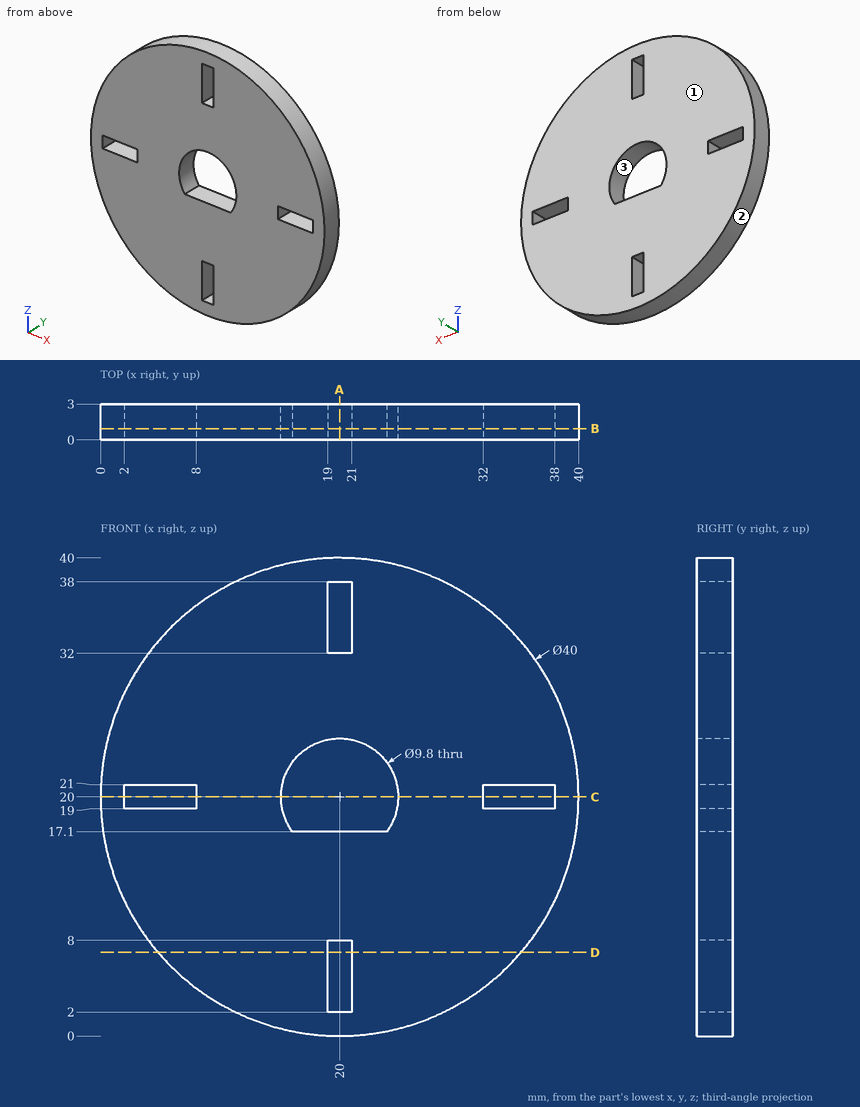
Job drawing, mm, ordinate dimensions from the low corner. One solid piece. Round coordinates to 2 decimals unless told otherwise and drop trailing zeros. Write each loop counter-clockwise with the first axis right and the second up, starting at its lowest first coordinate (ties: lowest second). Pieces come first, ordered by that corner, then holes.
1) Band-saw the part on C-C, the plane z = 20. List the corners of the cut face in (x, y), and give its area (3 significant figures).
2) Band-saw the part on A-A, the plane x = 20. List the corners of the cut face in (y, z).
3) Drill centre lines: probe 1 along Z at (x, y) = (20, 1.3); probe 2 along X at (y, z) = (2.8, 34); probe 3 along Z at (x, y) = (23.5, 0.1). Where is each one in solid material? Low to high.
4) Mould opens along X. For the marked faces 1, 2 and 3 say: +X half, -X half, draft (parallel to the pull), parting line (faces both ways), or undercut.
5) Pin check, flat tips, straight feed: pin 1 (0.9 mm diameter, centred on x = 5.5, y = 1, fed in from -Z); pin 2 (1.5 mm diameter, centred on x = 19, y = 0.5, fed in from -Z); pin 3 (1.5 mm diameter, centred on y = 1, z = 4, fed in from +X). Stop position of each tip, or through.
6) Band-saw the part on B-B, the plane y = 0.95. List the corners of the cut face in (x, z).
7) Band-saw the part on D-D, the plane z = 7. List the corners of the cut face in (x, y).
Ans:
1. outline: (0, 0) - (2, 0) - (2, 3) - (0, 3) - close; (8, 0) - (15.1, 0) - (15.1, 3) - (8, 3) - close; (24.9, 0) - (32, 0) - (32, 3) - (24.9, 3) - close; (38, 0) - (40, 0) - (40, 3) - (38, 3) - close
1. area: 54.6 mm2
2. outline: (0, 0) - (3, 0) - (3, 2) - (0, 2) - close; (0, 8) - (3, 8) - (3, 17.1) - (0, 17.1) - close; (0, 24.9) - (3, 24.9) - (3, 32) - (0, 32) - close; (0, 38) - (3, 38) - (3, 40) - (0, 40) - close
3. probe 1: z = 0 to 2, 8 to 17.1, 24.9 to 32, 38 to 40
3. probe 2: x = 5.72 to 19, 21 to 34.28
3. probe 3: z = 0.31 to 17.1, 23.43 to 39.69
4. face 1: draft
4. face 2: parting line
4. face 3: undercut
5. pin 1: stops at z = 5.77
5. pin 2: stops at z = 0
5. pin 3: stops at x = 32.94
6. outline: circle Ø40 at (20, 20); hole (2, 19) - (8, 19) - (8, 21) - (2, 21) - close; hole (16.05, 17.1) - (23.95, 17.1) arc R4.9 ccw (long way) to start; hole (19, 2) - (21, 2) - (21, 8) - (19, 8) - close; hole (19, 32) - (21, 32) - (21, 38) - (19, 38) - close; hole (32, 19) - (38, 19) - (38, 21) - (32, 21) - close
7. outline: (4.8, 0) - (19, 0) - (19, 3) - (4.8, 3) - close; (21, 0) - (35.2, 0) - (35.2, 3) - (21, 3) - close
